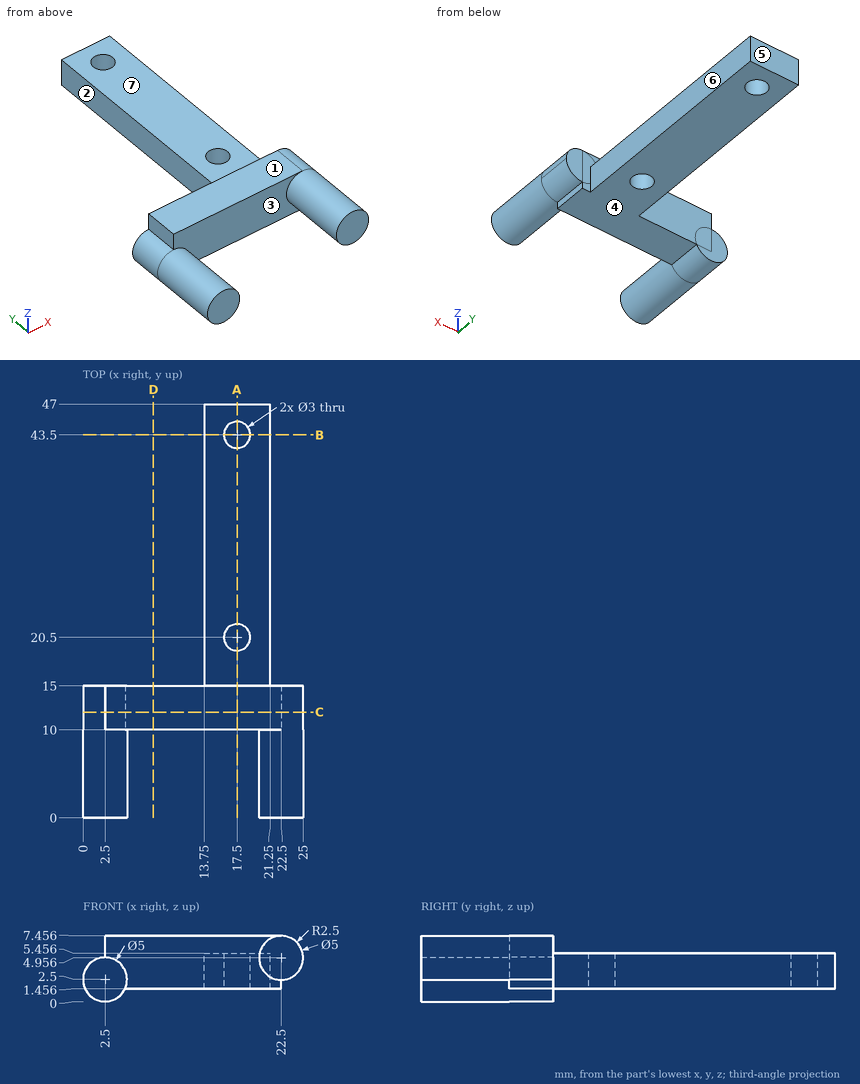
Input: dimensioned drawing with shaded views. Units: mm. Origin: part minimum x, y, z. A direction names the side the tool comes from. Coordinates: 2 decimals unless noted, no trailing zeros. Write each loop counter-clockwise with the first axis right and the second up, starting at its lowest first coordinate (ties: lowest second). Pieces come first, ordered by that corner, then holes. Notation, with made-up numbers: M -9,67.25 L 13,67.25 A20 ccw 13,95.25 Z; hole C -19,18.25 d5. An arc over 180 degrees is marked long. Answer as CSV lines item,"result". Start each with the question number.
Q1. Reachability of the marked faces 4, 5, 6 and 7 from +Z, -Z, +X, -X, +Y, -Y: full face, straight path, thin tool, end or side. Return the list, or none.
Q2. Cut plane A-A on x = 17.5. Return the cut outline in (y, z).
Q3. Mould query, pull axis X, two halves, no side actions, for the marked faces 1, 2 and 3. Classes: released by +X, released by -X, zero draft, split by the parting line, or undercut.
Q4. Cut plane C-C on y = 12. Return the cut outline in (x, z).
Q5. Cut plane D-D on x = 8. Return the cut outline in (y, z).
Q6. Cut plane B-B on y = 43.5. Return the cut outline in (x, z), then the cut area to 3 significant figures.
Q7. Line query: line 1 (Y direction, x = 17.5, z = 4.5); line 2 (Y direction, x = 16, z = 5.75); line 3 (Z direction, x = 7.25, y = 11). Output: solid intervals per line, ascending. Write a range as from..to.
Q8. Pin query (flat end, axial travel): P1, Ø2.5, axis at x = 20.5, z = 6, coming from the +Y side; P2, Ø1.5, axis at x = 7, z = 2.5, coming from the +Y side; P3, Ø8, axis at x = 19, y = 27.5, coming from the +Z side; P4, Ø2, axis at y = 26.5, z = 3, coming from the +X side. Return the tip coordinate at first contact, or that it passes through.
Findings below:
1,face 4,"-Z, +X, +Y, -Y"
1,face 5,"+Z, -Z, +X, -X, +Y"
1,face 6,"+Z, -Z, +X, +Y"
1,face 7,"+Z, +X, -X, +Y"
2,outline,"M 10,1.46 L 19,1.46 L 19,5.46 L 15,5.46 L 15,7.46 L 10,7.46 Z; M 22,1.46 L 42,1.46 L 42,5.46 L 22,5.46 Z; M 45,1.46 L 47,1.46 L 47,5.46 L 45,5.46 Z"
3,face 1,"zero draft"
3,face 2,"released by -X"
3,face 3,"undercut"
4,outline,"M 2.5,5 A2.5 ccw long 4.77,1.46 L 22.5,1.46 L 22.5,2.46 A2.5 ccw 22.5,7.46 L 2.5,7.46 Z"
5,outline,"M 10,1.46 L 15,1.46 L 15,7.46 L 10,7.46 Z"
6,outline,"M 13.75,1.46 L 16,1.46 L 16,5.46 L 13.75,5.46 Z; M 19,1.46 L 21.25,1.46 L 21.25,5.46 L 19,5.46 Z"
6,area,"18.0 mm2"
7,line 1,"y = 10..19, 22..42, 45..47"
7,line 2,"y = 10..15"
7,line 3,"z = 1.46..7.46"
8,P1,"stops at y = 47"
8,P2,"stops at y = 15"
8,P3,"stops at z = 5.46"
8,P4,"stops at x = 21.25"
